Part model, mm, in its own coordinate system. A direction names the side the tool comes from. Give positions to 0.01 mm unless a question says otherwise; leave off trailing zeros. Write each loop counter-clockwise with the first axis right and the second up, starting at its lowest first coordinate (ties: lowest second). Pieces come first, ordered by that corner, then holes. Notation, with made-up numbers: M 79,27 L 88,27 A28 cw 88,61 Z; hole C 49,69.5 d10. An arc over 180 degrees is marked long. Use CSV: the item, a comma, the result in double quotes. Start each with the question number.
Item 1: Which spindle directions (+Z, -Z, +X, -X, +Y, -Y) get a long thin tool onto all of the face, cutting with end or side? Do faces 1 (the flat face through (-32, 46.375, 2)), 2 (the flat face through (32, 46.375, 2)), 3 (the flat face through (32, -46.375, 2)), 4 (the flat face through (-32, -46.375, 2)), 5 (the flat face through (0, -51.375, 2)). Say none if no direction does.
Item 2: Cut at A-A (z = 0.8). Count the separate pieces of the cut face and the enclosed holes in it, then the cut area to 3 significant figures.
Item 3: Drill centre lines: line 1 (Y direction, x = 15, z = 0.6) (3 decimals); line 2 (Y direction, x = -24.5, z = 1.35) (3 decimals); line 3 (Y direction, x = 17, z = 0.4). Where is each one in solid material? Low to high. Write a range as [from, to].
Item 4: Cut at B-B (x = -34.5). List the corners of the cut face in (y, z) (3 decimals), then the cut area to 3 significant figures.
Item 5: Pin check, flat tips, straight feed: pin 1 (4 mm diameter, centred on x = -15.025, y = 50.975, fed in from -Z); pin 2 (1 mm diameter, centred on x = -20.5, z = 2.5, fed in from +Y); pin 3 (3 mm diameter, centred on x = 15.025, y = -47.025, fed in from -Z); pin 4 (1.1 mm diameter, centred on y = -48.5, z = 1, fed in from -X). Stop position of each tip, or through.
Item 6: Mould opens along Y. For faces 6 (the cylindrical face through (-13.5, 51.46, 1.5)), 7 (the flat face through (46.375, -1, 2)), 8 (the cylindrical face through (16.55, 51.46, 1.5)), 9 (the cylindrical face through (45.52, -45.47, 1.55)) say: released by +Y, released by -Y, zero draft, split by the parting line, or undercut.
from build123d import *

# Parameters (mm, degrees)
F0_W     = 37.75
F0_H     = 9
F0_R     = 1.6
F1_DEPTH = 3.05
F2_R     = 2
F3_R     = 3


with BuildPart() as f1:
    # F0 (on Top) → F1 (new body)
    with BuildSketch(Plane.XY):
        with BuildLine():
            Line((-18.875, 46.375), (-46.375, 46.375))
            Line((-46.375, 46.375), (-46.375, -46.375))
            Line((-46.375, -46.375), (-18.875, -46.375))
            Line((-18.875, -46.375), (-16.487019, -46.375))
            ThreePointArc((-16.487019, -46.375), (-15.025, -45.425), (-13.562981, -46.375))
            Line((-13.562981, -46.375), (13.562981, -46.375))
            ThreePointArc((13.562981, -46.375), (15.025, -45.425), (16.487019, -46.375))
            Line((16.487019, -46.375), (18.875, -46.375))
            Line((18.875, -46.375), (46.375, -46.375))
            Line((46.375, -46.375), (46.375, 46.375))
            Line((46.375, 46.375), (18.875, 46.375))
            Line((18.875, 46.375), (-18.875, 46.375))
        make_face()
        with BuildLine():
            Line((-16.487019, -46.375), (-18.875, -46.375))
            Line((-18.875, -46.375), (-18.875, -51.375))
            Line((-18.875, -51.375), (18.875, -51.375))
            Line((18.875, -51.375), (18.875, -46.375))
            Line((18.875, -46.375), (16.487019, -46.375))
            ThreePointArc((16.487019, -46.375), (16.590125, -46.692758), (16.625, -47.025))
            ThreePointArc((16.625, -47.025), (14.692758, -48.590125), (13.562981, -46.375))
            Line((13.562981, -46.375), (-13.562981, -46.375))
            ThreePointArc((-13.562981, -46.375), (-13.459875, -46.692758), (-13.425, -47.025))
            ThreePointArc((-13.425, -47.025), (-15.357242, -48.590125), (-16.487019, -46.375))
        make_face()
        with Locations((0, 50.875)):
            Rectangle(F0_W, F0_H)
        with Locations((-15.025, 50.975)):
            Circle(F0_R, mode=Mode.SUBTRACT)
        with Locations((15.025, 50.975)):
            Circle(F0_R, mode=Mode.SUBTRACT)
    extrude(amount=F1_DEPTH)

    # F2
    f2_edges = [f1.edges().sort_by_distance(p)[0] for p in [
        (18.875, 46.375, 1.525),
        (-18.875, 46.375, 1.525),
        (-18.875, -46.375, 1.525),
        (18.875, -46.375, 1.525),
        (-18.875, 55.375, 1.525),
        (18.875, 55.375, 1.525),
        (18.875, -51.375, 1.525),
        (-18.875, -51.375, 1.525),
    ]]
    fillet(f2_edges, radius=F2_R)

    # F3
    f3_edges = [f1.edges().sort_by_distance(p)[0] for p in [
        (-46.375, -46.375, 1.525),
        (46.375, -46.375, 1.525),
        (46.375, 46.375, 1.525),
        (-46.375, 46.375, 1.525),
    ]]
    fillet(f3_edges, radius=F3_R)


solid = f1.part
Worked answers:
1,face 1,"+Z, -Z, -X, +Y"
1,face 2,"+Z, -Z, +X, +Y"
1,face 3,"+Z, -Z, +X, -Y"
1,face 4,"+Z, -Z, -X, -Y"
1,face 5,"+Z, -Z, +X, -X, -Y"
2,separate pieces,"1"
2,enclosed holes,"4"
2,area,"9,090 mm^2"
3,line 1,"y = [-51.375, -48.625], [-45.425, 49.375], [52.575, 55.375]"
3,line 2,"y = [-46.375, 46.375]"
3,line 3,"y = [-51.37, 55.37]"
4,outline,"M -46.375,0 L 46.375,0 L 46.375,3.05 L -46.375,3.05 Z"
4,area,"283 mm^2"
5,pin 1,"stops at z = 0"
5,pin 2,"stops at y = 46.58"
5,pin 3,"passes through"
5,pin 4,"stops at x = -18.92"
6,face 6,"undercut"
6,face 7,"zero draft"
6,face 8,"undercut"
6,face 9,"released by -Y"
